Geometry check sheet. Reference: the model listing, model coordinates, mm. A direction names the side the tool comes from. Coordinates: 2 decimals unless noted, no trailing zeros. Order: outer loops, then holes, each group sorted by start corner. A loop starts at its lowest first (then second) coordinate and runs counter-clockwise, first axis right, second up. Notation, with made-up numbers: M 23,13.25 L 57,13.25 A25 ccw 57,28.25 Z; hole C -17.5,-24 d10. An arc over 180 degrees is marked long. Use CSV: the item, a comma, the result in double quotes. Start each with the question number.
```python
from build123d import *

# Parameters (mm, degrees)
CROQUIS1_R              = 2
CROQUIS1_R_2            = 4.05
CROQUIS1_R_3            = 12.5
SALIENTE_EXTRUIR1_DEPTH = 5
CROQUIS2_R              = 7.5
CROQUIS2_R_2            = 2.5
CROQUIS2_R_3            = 2
CORTAR_EXTRUIR1_DEPTH   = 10


with BuildPart() as part:
    # Croquis1 → Saliente-Extruir1 (new body)
    with BuildSketch(Plane(origin=(0, 0, 0), x_dir=(0, 0, -1), z_dir=(1, 0, 0))):
        with BuildLine():
            Line((10, 0), (60, 0))
            ThreePointArc((60, 0), (67.071067812, 2.928932188), (70, 10))
            Line((70, 10), (70, 60))
            ThreePointArc((70, 60), (67.071067812, 67.071067812), (60, 70))
            Line((60, 70), (60, 80))
            ThreePointArc((60, 80), (57.071067812, 87.071067812), (50, 90))
            Line((50, 90), (20, 90))
            ThreePointArc((20, 90), (12.928932188, 87.071067812), (10, 80))
            Line((10, 80), (10, 70))
            ThreePointArc((10, 70), (2.928932188, 67.071067812), (0, 60))
            Line((0, 60), (0, 10))
            ThreePointArc((0, 10), (2.928932188, 2.928932188), (10, 0))
        make_face()
        with Locations((7, 63)):
            Circle(CROQUIS1_R, mode=Mode.SUBTRACT)
        with Locations((63, 63)):
            Circle(CROQUIS1_R, mode=Mode.SUBTRACT)
        with Locations((63, 7)):
            Circle(CROQUIS1_R, mode=Mode.SUBTRACT)
        with Locations((7, 7)):
            Circle(CROQUIS1_R, mode=Mode.SUBTRACT)
        with Locations((53.05, 31.84)):
            Circle(CROQUIS1_R_2, mode=Mode.SUBTRACT)
        with Locations((35, 35)):
            Circle(CROQUIS1_R_3, mode=Mode.SUBTRACT)
    extrude(amount=SALIENTE_EXTRUIR1_DEPTH)

    # Croquis2 → Cortar-Extruir1 (cut)
    with BuildSketch(Plane(origin=(5, 0, 0), x_dir=(0, 0, -1), z_dir=(1, 0, 0))):
        with Locations((15, 0)):
            Circle(CROQUIS2_R)
        with Locations((50, 58)):
            Circle(CROQUIS2_R_2)
        with Locations((52, 83)):
            Circle(CROQUIS2_R_3)
        with Locations((34, 83)):
            Circle(CROQUIS2_R_3)
    extrude(amount=-CORTAR_EXTRUIR1_DEPTH, mode=Mode.SUBTRACT)


solid = part.part
```
1) Section check A-A on x = 3.3. State how many separate pieces and enclosed holes the cut face has, then the cut area to 3 significant figures.
2) Section check C-C on z = -43.5. Record the boundary of the cut face in (x, y), then the cut area to 3 significant figures.
3) Set-up check for faces 4 (the face through (2.535, 7.493, -15.321)), 5 (the face through (2, 75, -60)): record each of +Z, -Z, +X, -X, +Y, -Y from which the full face is reachable in a straight line by a thin tool's end or side.
4) Gauge pin test, flat ends, axial feed: P1, Ø2.5, axis at y = 63, z = -7, coming from the -X side; P2, Ø4.5, axis at y = 83, z = -52, coming from the +X side; P3, Ø2, axis at x = 1, z = -7, coming from the +Y side. Record the tip position at first contact, or that the pin passes through.
5) Draft check along Z on faces 1 (the face through (5, 46, -42)), 2 (the face through (2, 35, 0)), 3 (the face through (2, 65, -7)). Enter one of: +Z half, -Z half, draft (parallel to the pull), parting line (faces both ways), or undercut.
6) Section check D-D on y = 83. Record the boundary of the cut face in (x, z).
7) Section check B-B on y = 58. Record the boundary of the cut face in (x, z), then the cut area to 3 significant figures.
8) Material ranges on line 1 along Y through (x, z) = (2.2, -7); line 2 along Y through (x, z) = (3.2, -52); line 3 along Y through (x, z) = (1.3, -51.5), recorded low to high.
Results are:
1,separate pieces,"1"
1,enclosed holes,"9"
1,area,"5,050 mm²"
2,outline,"M 0,0 L 5,0 L 5,25.83 L 0,25.83 Z; M 0,44.17 L 5,44.17 L 5,90 L 0,90 Z"
2,area,"358 mm²"
3,face 4,"+X, -X, -Y"
3,face 5,"-Z, +X, -X, +Y"
4,P1,"passes through"
4,P2,"stops at x = 5"
4,P3,"stops at y = 69.8"
5,face 1,"draft"
5,face 2,"+Z half"
5,face 3,"undercut"
6,outline,"M 0,-59.54 L 5,-59.54 L 5,-54 L 0,-54 Z; M 0,-50 L 5,-50 L 5,-36 L 0,-36 Z; M 0,-32 L 5,-32 L 5,-10.46 L 0,-10.46 Z"
7,outline,"M 0,-70 L 5,-70 L 5,-52.5 L 0,-52.5 Z; M 0,-47.5 L 5,-47.5 L 5,0 L 0,0 Z"
7,area,"325 mm²"
8,line 1,"y = 0.46 to 5, 9 to 61, 65 to 69.54"
8,line 2,"y = 0 to 27.93, 35.75 to 56.5, 59.5 to 81, 85 to 89.8"
8,line 3,"y = 0 to 28.1, 35.58 to 56, 60 to 81.06, 84.94 to 89.89"
